The model under review builds one solid part; all positions refer to its coordinate system, in mm. Face numbers are marked on the shaded views. Coordinates: 2 decimals unless noted, no trailing zeros. Order: outer loops, then holes, each group sorted by start corner. A loop starts at its lowest first (then second) coordinate and runs counter-clockwise, first axis right, second up. Notation, with made-up numbers: (-33.5, 69) -> (24.5, 69) arc R16 ccw to (24.5, 84) -> close; hole circle Ø9 at (46.25, -13.75). An arc over 180 degrees is marked (long way). Use one line per item in the form item = value. Start each with the question number.
(1) Take a section at A-A (y = 0). State the section outline as (x, z) points (3 decimals), then the cut area to 3 significant figures.
(2) Mouldability with a two-part tool opening along X and no side actions: class the marked faces 1, 2, 3 and 4 as +X half, -X half, draft (parallel to the pull), parting line (faces both ways), or undercut.
(3) Take a section at B-B (x = 39). State the section outline as (y, z) points, then the cut area to 3 significant figures.
(4) Insertion check: pin 1 Ø12 at (x, z) = (17, 34.5) entering from +Y; pin 2 Ø5 at (y, z) = (-14.5, 42.5) entering from -X; pin 3 Ø10 at (y, z) = (-20.5, 8.5) entering from +X. Each pin has a flat end and moves straight along its axis. Give the tip position at first contact, or say it passes through.
(5) Wall thickness on line 1 along X through (y, z) = (-0.5, 39.5); line 2 along X through (y, z) = (1.5, 24.5); line 3 along Y through (x, z) = (0, 14) (3 decimals): over which ranges is each line inside the solid? List them lowest first.
(6) Take a section at C-C (z = 36). State the section outline as (x, y) points (3 decimals), then the cut area to 3 significant figures.
(7) Take a section at D-D (x = 0). State the section outline as (y, z) points (3 decimals).
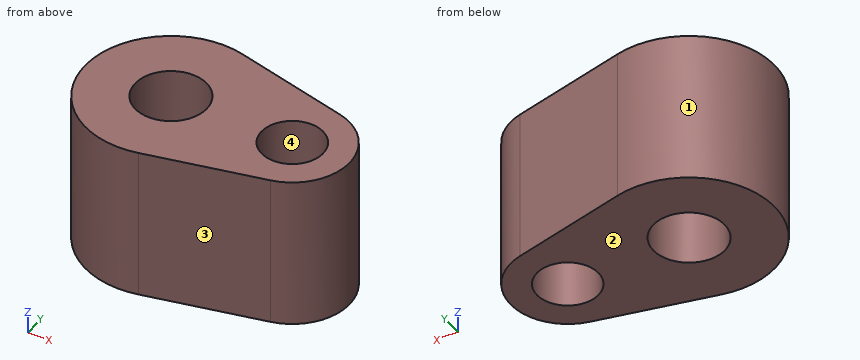
```python
from build123d import *

# Parameters (mm, degrees)
F0_R        = 11.915187
F0_R_2      = 10.259899
F1_DEPTH    = 25.4
F1_FACE_R   = 11.915187
F1_FACE_R_2 = 10.259899
F2_DEPTH    = 12.7
F3_DEPTH    = 25.4


with BuildPart() as f1:
    # F0 (on Top) → F1 (new body)
    with BuildSketch(Plane.XY):
        with BuildLine():
            Line((45.557722, 18.532589), (6.614583, 27.798883))
            ThreePointArc((6.614583, 27.798883), (-28.575, 0), (6.614583, -27.798883))
            Line((6.614583, -27.798883), (45.557722, -18.532589))
            ThreePointArc((45.557722, -18.532589), (60.198, 0), (45.557722, 18.532589))
        make_face()
        Circle(F0_R, mode=Mode.SUBTRACT)
        with Locations((41.148, 0)):
            Circle(F0_R_2, mode=Mode.SUBTRACT)
    extrude(amount=F1_DEPTH)

    # F1_face (on face) → F2 (join)
    with BuildSketch(Plane(origin=(12.189133, 0, 25.4), x_dir=(1, 0, 0), z_dir=(0, 0, 1))):
        with BuildLine():
            Line((-5.57455, -27.798883), (33.368589, -18.532589))
            ThreePointArc((33.368589, -18.532589), (48.008867, 0), (33.368589, 18.532589))
            Line((33.368589, 18.532589), (-5.57455, 27.798883))
            ThreePointArc((-5.57455, 27.798883), (-40.764133, 0), (-5.57455, -27.798883))
        make_face()
        with Locations((-12.189133, 0)):
            Circle(F1_FACE_R, mode=Mode.SUBTRACT)
        with Locations((28.958867, 0)):
            Circle(F1_FACE_R_2, mode=Mode.SUBTRACT)
    extrude(amount=-F2_DEPTH)

    # F1_face (on face) → F3 (join)
    with BuildSketch(Plane(origin=(12.189133, 0, 25.4), x_dir=(1, 0, 0), z_dir=(0, 0, 1))):
        with BuildLine():
            Line((-5.57455, -27.798883), (33.368589, -18.532589))
            ThreePointArc((33.368589, -18.532589), (48.008867, 0), (33.368589, 18.532589))
            Line((33.368589, 18.532589), (-5.57455, 27.798883))
            ThreePointArc((-5.57455, 27.798883), (-40.764133, 0), (-5.57455, -27.798883))
        make_face()
        with Locations((-12.189133, 0)):
            Circle(F1_FACE_R, mode=Mode.SUBTRACT)
        with Locations((28.958867, 0)):
            Circle(F1_FACE_R_2, mode=Mode.SUBTRACT)
    extrude(amount=F3_DEPTH)


solid = f1.part
```
Findings:
q1.outline = (-28.575, 0) -> (-11.915, 0) -> (-11.915, 50.8) -> (-28.575, 50.8) -> close; (11.915, 0) -> (30.888, 0) -> (30.888, 50.8) -> (11.915, 50.8) -> close; (51.408, 0) -> (60.198, 0) -> (60.198, 50.8) -> (51.408, 50.8) -> close
q1.area = 2,260 mm²
q2.face_1 = parting line
q2.face_2 = draft
q2.face_3 = +X half
q2.face_4 = undercut
q3.outline = (-20.09, 0) -> (-10.03, 0) -> (-10.03, 50.8) -> (-20.09, 50.8) -> close; (10.03, 0) -> (20.09, 0) -> (20.09, 50.8) -> (10.03, 50.8) -> close
q3.area = 1,020 mm²
q4.pin_1 = 26.76
q4.pin_2 = -25.93
q4.pin_3 = 52.22
q5.line_1 = -28.57 to -11.9, 11.9 to 30.9, 51.4 to 60.19
q5.line_2 = -28.54 to -11.82, 11.82 to 31, 51.3 to 60.14
q5.line_3 = -28.575 to -11.915, 11.915 to 28.575
q6.outline = (6.615, -27.799) -> (45.558, -18.533) arc R19.05 ccw to (45.558, 18.533) -> (6.615, 27.799) arc R28.575 ccw (long way) to start; hole circle Ø23.83 at (0, 0); hole circle Ø20.52 at (41.148, 0)
q6.area = 3,090 mm²
q7.outline = (-28.575, 0) -> (-11.915, 0) -> (-11.915, 50.8) -> (-28.575, 50.8) -> close; (11.915, 0) -> (28.575, 0) -> (28.575, 50.8) -> (11.915, 50.8) -> close
